from build123d import *

# Parameters (mm, degrees)
SKETCH_1_W                   = 196
SKETCH_1_H                   = 246
EXTRUDE_1_DEPTH              = 22
HOLE_WIZARD_M101_D           = 11
HOLE_WIZARD_M101_CBORE_D     = 18
HOLE_WIZARD_M101_CBORE_DEPTH = 13
HOLE_WIZARD_M221_D           = 26
HOLE_WIZARD_M801_D           = 90
HOLE_WIZARD_M801_DEPTH       = 4


with BuildPart() as part:
    # Эскиз1 → Бобышка-Вытянуть1 (new body)
    with BuildSketch(Plane.XY.offset(22)):
        Rectangle(SKETCH_1_W, SKETCH_1_H)
    extrude(amount=-EXTRUDE_1_DEPTH)

    # Цековка для  болта с шестигранной головкой M101 (through all)
    with Locations(Plane.XY.offset(22)):
        with Locations((50, 77), (50, -77), (-50, 77), (-50, -77)):
            CounterBoreHole(HOLE_WIZARD_M101_D / 2, HOLE_WIZARD_M101_CBORE_D / 2, HOLE_WIZARD_M101_CBORE_DEPTH)

    # Отверстие с зазором M221 (through all)
    with Locations(Plane.XY.offset(22)):
        with Locations((76, 77), (76, -77), (-76, -77), (-76, 77)):
            Hole(HOLE_WIZARD_M221_D / 2)

    # Отверстие с зазором M801
    with Locations(Plane.XY.offset(22)):
        with Locations((0, 0)):
            Hole(HOLE_WIZARD_M801_D / 2, depth=HOLE_WIZARD_M801_DEPTH)


solid = part.part
Verification items for the finished model (mm, model axes). A direction names the side the tool comes from. Give positions to 0.01 mm unless a question says otherwise; leave off trailing zeros. Loops run counter-clockwise (first coordinate to the right, second up) from the corner with the lowest first, then second, coordinate; pieces in that order, holes last. Notation, with made-up numbers: (34, 86.5) - (45, 86.5) arc R21 cw to (45, 91.5) - close; hole circle Ø5 at (10.25, 78). An arc over 180 degrees is marked (long way). Write each question's results on one line, items separated by ' | '.
1) Material ranges on L1, parallel to Y at x = -50, z = 4.5; L2, parallel to Y at x = 50, z = 17.75; L3, parallel to X at y = -76.5, z = 4.5, recorded low to high. Write a range as from..to.
Solution:
L1: -123..-82.5, -71.5..71.5, 82.5..123 | L2: -123..-86, -68..68, 86..123 | L3: -98..-88.99, -63.01..-55.48, -44.52..44.52, 55.48..63.01, 88.99..98
2) Tool access check on faces 4 (the cylindrical face through (-63.013, 77.572, 10.846)), 5 (the cylindrical face through (-51.951, 68.214, 15.591)). Record the directions out of +Z, -Z, +X, -X, +Y, -Y that give a thin tool (end or side, any length) a straight path to the whole face; none if there is none.
Solution:
face 4: +Z, -Z | face 5: +Z
3) Sectioned sample at B-B on y = -77. Record the boundary of the cut face in (x, z), plus the area to 3 significant figures.
Solution:
outline: (-98, 0) - (-89, 0) - (-89, 22) - (-98, 22) - close; (-63, 0) - (-55.5, 0) - (-55.5, 9) - (-59, 9) - (-59, 22) - (-63, 22) - close; (-44.5, 0) - (44.5, 0) - (44.5, 9) - (41, 9) - (41, 22) - (-41, 22) - (-41, 9) - (-44.5, 9) - close; (55.5, 0) - (63, 0) - (63, 22) - (59, 22) - (59, 9) - (55.5, 9) - close; (89, 0) - (98, 0) - (98, 22) - (89, 22) - close | area: 2,500 mm2
4) Sectioned sample at D-D on x = 0. Record the boundary of the cut face in (y, z), plus the area to 3 significant figures.
Solution:
outline: (-123, 0) - (123, 0) - (123, 22) - (45, 22) - (45, 18) - (-45, 18) - (-45, 22) - (-123, 22) - close | area: 5,050 mm2
5) Sectioned sample at C-C on z = 3.5. Count the separate pieces of the cut face and the enclosed holes in it, plus the area to 3 significant figures.
Solution:
separate pieces: 1 | enclosed holes: 8 | area: 45,700 mm2
6) Depth check by flat-ended pin: P1, Ø5.5, axis at x = 51.5, y = -74, coming from the +Z side. Enter the tip coordinate at first touch or a pass-through.
Solution:
P1: z = 9
7) Mould release check, pull along Y, two halves, no side actions. Record for faces 1 (the flat face through (-1, -123, 11)), 2 (the cylindrical face through (-45.95, 80.72, 4.44)), 3 (the flat face through (42, 29, 22)): pulls with the +Y half, pulls with the -Y half, needs draft (parallel to the pull), parting line crosses it, or undercut.
Solution:
face 1: pulls with the -Y half | face 2: undercut | face 3: needs draft
8) Sectioned sample at A-A on x = -50. Record the boundary of the cut face in (y, z).
Solution:
outline: (-123, 0) - (-82.5, 0) - (-82.5, 9) - (-86, 9) - (-86, 22) - (-123, 22) - close; (-71.5, 0) - (71.5, 0) - (71.5, 9) - (68, 9) - (68, 22) - (-68, 22) - (-68, 9) - (-71.5, 9) - close; (82.5, 0) - (123, 0) - (123, 22) - (86, 22) - (86, 9) - (82.5, 9) - close
